```python
from build123d import *

# Parameters (mm, degrees)
SKETCH_1_R          = 2.2
EXTRUDE_2_DEPTH     = 6
SKETCH_2_R          = 1.6
CUT_EXTRUDE_2_DEPTH = 26
SKETCH_3_W          = 22.036316786
SKETCH_3_H          = 24
CUT_EXTRUDE_3_DEPTH = 2
CUT_EXTRUDE_4_DEPTH = 27
CUT_EXTRUDE_7_DEPTH = 24
EXTRUDE_4_DEPTH     = 24
SKETCH_9_W          = 6
SKETCH_9_H          = 5.089389346
CUT_EXTRUDE_8_DEPTH = 24


with BuildPart() as part:
    # 草图1 → 凸台-拉伸2 (new body)
    with BuildSketch(Plane(origin=(0, 0, 0), x_dir=(1, 0, 0), z_dir=(0, 1, 0))):
        Polygon((4.305555556, 9.700757576), (-25.694444444, 9.700757576), (-25.694444444, -14.299242424), (4.305555556, -14.299242424), (4.305555556, -10.299242424), (-5.694444444, -10.299242424), (-5.694444444, -4.299242424), (4.305555556, -4.299242424), align=None)
        with Locations(Location((-12.043257461, -2.299242424, 0), (0, 0, 270))):
            Circle(SKETCH_1_R, mode=Mode.SUBTRACT)
        with Locations(Location((-20.043257461, 1.200757576, 0), (0, 0, 270))):
            Circle(SKETCH_1_R, mode=Mode.SUBTRACT)
        with Locations(Location((-12.043257461, 4.700757576, 0), (0, 0, 270))):
            Circle(SKETCH_1_R, mode=Mode.SUBTRACT)
    extrude(amount=EXTRUDE_2_DEPTH)

    # 草图2 → 切除-拉伸2 (cut)
    with BuildSketch(Plane.XY.offset(14.299242424)):
        with Locations((2.152777778, 3)):
            Circle(SKETCH_2_R)
    extrude(amount=-CUT_EXTRUDE_2_DEPTH, mode=Mode.SUBTRACT)

    # 草图3 → 切除-拉伸3 (cut)
    with BuildSketch(Plane.XZ):
        with Locations((-14.676286051, 2.299242424)):
            Rectangle(SKETCH_3_W, SKETCH_3_H)
    extrude(amount=-CUT_EXTRUDE_3_DEPTH, mode=Mode.SUBTRACT)

    # 草图4 → 切除-拉伸4 (cut)
    with BuildSketch(Plane.XY.offset(14.299242424)):
        Polygon((-1.100112358, 0), (-3.658127658, 2), (-3.658127658, 0), align=None)
    extrude(amount=-CUT_EXTRUDE_4_DEPTH, mode=Mode.SUBTRACT)

    # 草图5 → 切除-拉伸7 (cut)
    with BuildSketch(Plane(origin=(0, 0, -9.700757576), x_dir=(-1, 0, 0), z_dir=(0, 0, -1))):
        with BuildLine():
            Line((-2.152777778, 0), (-4.305555556, 0))
            Line((-4.305555556, 0), (-4.305555556, 0.910610654))
            ThreePointArc((-4.305555556, 0.910610654), (-3.32150186, 0.237015378), (-2.152777778, 0))
        make_face()
    extrude(amount=-CUT_EXTRUDE_7_DEPTH, mode=Mode.SUBTRACT)

    # 草图8 → 凸台-拉伸4 (add)
    with BuildSketch(Plane(origin=(0, 0, -9.700757576), x_dir=(-1, 0, 0), z_dir=(0, 0, -1))):
        with BuildLine():
            ThreePointArc((-4.305555556, 0.910610654), (-4.932915664, 1.872687562), (-5.152777778, 3))
            Line((-5.152777778, 3), (-5.152777778, 6))
            Line((-5.152777778, 6), (-4.305555556, 6))
            Line((-4.305555556, 6), (-4.305555556, 0.910610654))
        make_face()
    extrude(amount=-EXTRUDE_4_DEPTH)

    # 草图9 → 切除-拉伸8 (cut)
    with BuildSketch(Plane.ZY.offset(-4.305555556)):
        with Locations((7.299242424, 3.455305327)):
            Rectangle(SKETCH_9_W, SKETCH_9_H)
    extrude(amount=-CUT_EXTRUDE_8_DEPTH, mode=Mode.SUBTRACT)


solid = part.part
```
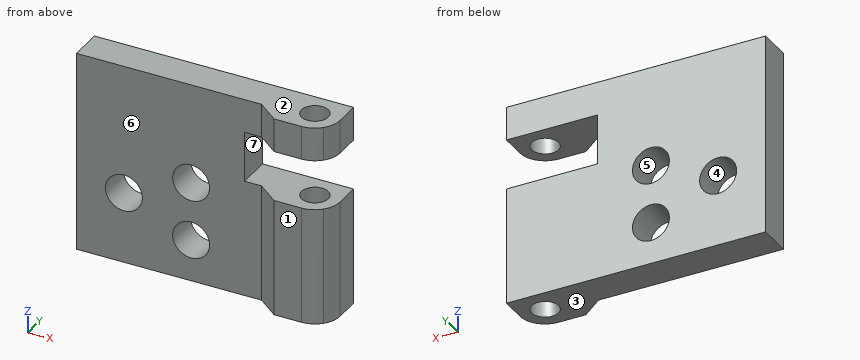
For this review, take the finished solid that the model builds, in its own axes (mm). Face numbers are marked on the shaded views. A direction names the side the tool comes from. Round coordinates to 2 decimals unless told otherwise and drop trailing zeros. Write each loop counter-clockwise with the first axis right and the second up, starting at its lowest first coordinate (ties: lowest second). Pieces come first, ordered by that corner, then holes. Notation, with made-up numbers: (14.25, -8.5) - (51.25, -8.5) arc R10 ccw to (51.25, 2.5) - close; hole circle Ø5 at (27, -17.5). An arc over 180 degrees is marked (long way). Answer as a JSON object with one key per item and string values.
1. Draft analysis for pull direction Z (two halves, no side actions). For the marked faces 1, 2, 3 and 4, state which applies: +Z half, -Z half, draft (parallel to the pull), parting line (faces both ways), or undercut.
Response values:
{"face 1": "draft", "face 2": "+Z half", "face 3": "-Z half", "face 4": "undercut"}
2. We need section C-C on x = -19.5. Give the boundary of the cut face in (y, z).
Response values:
{"outline": "(2, -9.7) - (6, -9.7) - (6, -3.33) - (2, -3.33) - close; (2, 0.93) - (6, 0.93) - (6, 14.3) - (2, 14.3) - close"}
3. We need section B-B on y = 4.2. Give the boundary of the cut face in (x, z).
Response values:
{"outline": "(-25.69, -9.7) - (1.09, -9.7) - (1.09, 4.3) - (-5.69, 4.3) - (-5.69, 10.3) - (1.09, 10.3) - (1.09, 14.3) - (-25.69, 14.3) - close; (3.21, -9.7) - (5.15, -9.7) - (5.15, 4.3) - (3.21, 4.3) - close; (3.21, 10.3) - (5.15, 10.3) - (5.15, 14.3) - (3.21, 14.3) - close; hole circle Ø4.4 at (-20.04, -1.2); hole circle Ø4.4 at (-12.04, -4.7); hole circle Ø4.4 at (-12.04, 2.3)"}
4. To check wall thickness, follow line 1 along Z through (x, y) = (1, 0.5); line 2 along Z through (x, y) = (-12.5, 2.5); line 3 along X through (y, z) = (3.75, 3.5). State the ranges of each line that lie inside material, in increasing order.
Response values:
{"line 1": "z = -9.7 to 4.3, 10.3 to 14.3", "line 2": "z = -9.7 to -6.85, -2.55 to 0.15, 4.45 to 14.3", "line 3": "x = -25.69 to -13.89, -10.2 to 0.74, 3.57 to 5.15"}
5. Tool access review of the marked faces 5, 6 and 7: name each direction out of +Z, -Z, +X, -X, +Y, -Y from which nothing blocks a thin tool from reaching the whole face with its end or side.
Response values:
{"face 5": "+Y, -Y", "face 6": "+Z, -Z, -X, -Y", "face 7": "+X, +Y, -Y"}
6. For pin 1 Ø5 at (x, z) = (-12.04, 2.3) entering from -Y; pin 2 Ø1.2 at (y, z) = (4.5, 7) entering from +X; pin 3 Ø12 at (x, z) = (-7.5, -5) entering from -Y, all flat-tipped, find the tip position at first contact; note any pin that passes through.
Response values:
{"pin 1": "stops at y = 2", "pin 2": "stops at x = -5.69", "pin 3": "stops at y = 0.31"}
7. We need section A-A on z = -6. Give the boundary of the cut face in (x, y).
Response values:
{"outline": "(-25.69, 2) - (-13.82, 2) - (-13.82, 6) - (-25.69, 6) - close; (-10.27, 2) - (-3.66, 2) - (-1.1, 0) - (2.15, 0) arc R3 ccw to (5.15, 3) - (5.15, 6) - (-10.27, 6) - close; hole circle Ø3.2 at (2.15, 3)"}
8. We need section D-D on z = 8.75. Give the boundary of the cut face in (x, y), then the cut area to 3 significant figures.
Response values:
{"outline": "(-25.69, 2) - (-5.69, 2) - (-5.69, 6) - (-25.69, 6) - close", "area": "80.0 mm2"}
